from build123d import *

# Parameters (mm, degrees)
F0_W     = 35
F0_H     = 20
F1_DEPTH = 10
F2_W     = 23
F2_H     = 13
F3_DEPTH = 10
F4_W     = 33
F4_H     = 13
F5_DEPTH = 4.5
F6_R     = 1.125
F6_W     = 1.5
F6_H     = 5
F7_DEPTH = 5.5
F8_R     = 1.125
F9_DEPTH = 1
F10_R    = 0.5


with BuildPart() as f1:
    # F0 (on Top) → F1 (new body)
    with BuildSketch(Plane.XY):
        Rectangle(F0_W, F0_H)
    extrude(amount=-F1_DEPTH)

    # F2 (on Top) → F3 (cut, through all)
    with BuildSketch(Plane.XY):
        Rectangle(F2_W, F2_H)
    extrude(amount=-F3_DEPTH, mode=Mode.SUBTRACT)

    # F4 (on Top) → F5 (cut)
    with BuildSketch(Plane.XY):
        Rectangle(F4_W, F4_H)
    extrude(amount=-F5_DEPTH, mode=Mode.SUBTRACT)

    # F6 (on face) → F7 (cut, through all)
    with BuildSketch(Plane.XY.offset(-4.5)):
        with Locations((-14.5, 0)):
            Circle(F6_R)
        with Locations((14.5, 0)):
            Circle(F6_R)
        with Locations((-12.25, 0)):
            Rectangle(F6_W, F6_H)
        with Locations((12.25, 0)):
            Rectangle(F6_W, F6_H)
    extrude(amount=-F7_DEPTH, mode=Mode.SUBTRACT)

    # F8 (on face) → F9 (cut)
    with BuildSketch(Plane(origin=(0, 0, -10), x_dir=(1, 0, 0), z_dir=(0, 0, -1))):
        Polygon((-15.943375673, -2.5), (-13.056624327, -2.5), (-13, -2.4019237886), (-13, 2.4019237886), (-13.056624327, 2.5), (-15.943375673, 2.5), (-17.3867513459, 0), align=None)
        with Locations((-14.5, 0)):
            Circle(F8_R, mode=Mode.SUBTRACT)
        Polygon((13, 2.4019237886), (13, -2.4019237886), (13.056624327, -2.5), (15.943375673, -2.5), (17.3867513459, 0), (15.943375673, 2.5), (13.056624327, 2.5), align=None)
        with Locations((14.5, 0)):
            Circle(F8_R, mode=Mode.SUBTRACT)
    extrude(amount=-F9_DEPTH, mode=Mode.SUBTRACT)

    # F10
    f10_edges = [f1.edges().sort_by_distance(p)[0] for p in [
        (-11.5, 4.5, -10),
        (-11.5, -4.5, -10),
        (0, -6.5, -10),
        (0, 6.5, -10),
        (11.5, 4.5, -10),
        (11.5, -4.5, -10),
        (11.5, -4.5, -4.5),
        (11.5, 4.5, -4.5),
        (-11.5, -4.5, -4.5),
        (-11.5, 4.5, -4.5),
    ]]
    fillet(f10_edges, radius=F10_R)


solid = f1.part
Model file for the job. Use its own axes, mm. A direction names the side the tool comes from. Give positions to 0.01 mm unless a question says otherwise; leave off trailing zeros. Loops run counter-clockwise (first coordinate to the right, second up) from the corner with the lowest first, then second, coordinate; pieces in that order, holes last.
1) Wall check: line 1 (X direction, y = 0, z = -6) (3 decimals); line 2 (X direction, y = 4, z = -7.75); line 3 (Y direction, x = 6.5, z = -0.25). Give the ranges that are in metal, low to high.
2) Saw through at C-C (z = -6). Write the cut outline in (x, y) (3 decimals), plus the area to 3 significant figures.
3) Saw through at A-A (y = -5). Write the cut outline in (x, z).
4) Saw through at D-D (z = -3.75). Write the cut outline in (x, y).
5) Flat gauge pins, fed straight in: pin 1 Ø1.5 at (x, y) = (1.5, -4) entering from -Z; pin 2 Ø3.5 at (x, y) = (-15, -0.5) entering from -Z; pin 3 Ø2 at (x, y) = (-14, 0.5) entering from +Z. Where does each tip first touch, or does it go through?
6) Pull direction X, two halves, no side cores. Call faces 3 (the flat face through (17.5, 0, -5)), 4 (the flat face through (-11.5, -5, -7)), 5 (the flat face through (0, 7, 0)): +X half, -X half, draft (parallel to the pull), parting line (faces both ways), or undercut.
7) Tool access for faces 1 (the flat face through (-14.5, 2.5, -9.5)), 2 (the flat face through (-13, 0, -7)): list every direction of +Z, -Z, +X, -X, +Y, -Y with a clear straight run to the whole face (end or side of a thin tool).
8) Saw through at B-B (x = 2). Write the cut outline in (y, z).
Answer block:
1. line 1: x = -17.5 to -15.625, -13.375 to -13, 13 to 13.375, 15.625 to 17.5
1. line 2: x = -17.5 to -11.5, 11.5 to 17.5
1. line 3: y = -10 to -6.5, 6.5 to 10
2. outline: (-17.5, -10) - (17.5, -10) - (17.5, 10) - (-17.5, 10) - close; hole circle Ø2.25 at (-14.5, 0); hole (-13, -2.5) - (-11.5, -2.5) - (-11.5, -6.5) - (11.5, -6.5) - (11.5, -2.5) - (13, -2.5) - (13, 2.5) - (11.5, 2.5) - (11.5, 6.5) - (-11.5, 6.5) - (-11.5, 2.5) - (-13, 2.5) - close; hole circle Ø2.25 at (14.5, 0)
2. area: 378 mm2
3. outline: (-17.5, -10) - (-12, -10) arc R0.5 ccw to (-11.5, -9.5) - (-11.5, -5) arc R0.5 ccw to (-12, -4.5) - (-16.5, -4.5) - (-16.5, 0) - (-17.5, 0) - close; (11.5, -9.5) arc R0.5 ccw to (12, -10) - (17.5, -10) - (17.5, 0) - (16.5, 0) - (16.5, -4.5) - (12, -4.5) arc R0.5 ccw to (11.5, -5) - close
4. outline: (-17.5, -10) - (17.5, -10) - (17.5, 10) - (-17.5, 10) - close; hole (-16.5, -6.5) - (16.5, -6.5) - (16.5, 6.5) - (-16.5, 6.5) - close
5. pin 1: passes through
5. pin 2: stops at z = -9
5. pin 3: stops at z = -4.5
6. face 3: +X half
6. face 4: undercut
6. face 5: draft
7. face 1: -Z
7. face 2: +Z, -Z
8. outline: (-10, -10) - (-7, -10) arc R0.5 ccw to (-6.5, -9.5) - (-6.5, 0) - (-10, 0) - close; (6.5, -9.5) arc R0.5 ccw to (7, -10) - (10, -10) - (10, 0) - (6.5, 0) - close
